from build123d import *

# Parameters (mm, degrees)
SKETCH_1_W      = 16.85
SKETCH_1_H      = 16.85
EXTRUDE_1_DEPTH = 4
SHELL_1_T       = -1.5
FILLET_1_R      = 1


with BuildPart() as part:
    # 草图1 → 凸台-拉伸1 (new body)
    with BuildSketch(Plane(origin=(0, 0, 0), x_dir=(1, 0, 0), z_dir=(0, 1, 0))):
        Rectangle(SKETCH_1_W, SKETCH_1_H)
    extrude(amount=EXTRUDE_1_DEPTH)

    # 抽壳1
    shell_1_openings = [part.faces().sort_by_distance(p)[0] for p in [
        (0, 0, 0),
    ]]
    offset(amount=SHELL_1_T, openings=shell_1_openings, kind=Kind.INTERSECTION)

    # 草图2 → 切除-旋转5 (revolve, cut)
    with BuildSketch(Plane.XY):
        with BuildLine():
            Line((0, 164), (0, 3))
            ThreePointArc((0, 3), (80.5, 83.5), (0, 164))
        make_face()
    revolve(axis=Axis((0, 0, 0), (0, 1, 0)), mode=Mode.SUBTRACT)

    # 圆角1
    fillet_1_edges = [part.edges().sort_by_distance(p)[0] for p in [
        (8.425, 1.943314789, 8.425),
        (-8.425, 1.943314789, 8.425),
        (0, 3.442087368, 8.425),
        (-8.425, 1.943314789, -8.425),
        (8.425, 1.943314789, -8.425),
        (0, 3.442087368, -8.425),
        (8.425, 3.553300166, 4.218359953),
        (-8.425, 3.442087368, 0),
    ]]
    fillet(fillet_1_edges, radius=FILLET_1_R)


solid = part.part
For this review, take the finished solid that the model builds, in its own axes (mm). A direction names the side the tool comes from. Give positions to 0.01 mm unless a question says otherwise; leave off trailing zeros. Loops run counter-clockwise (first coordinate to the right, second up) from the corner with the lowest first, then second, coordinate; pieces in that order, holes last.
Item 1: Draft analysis for pull direction X (two halves, no side actions). For faces 1 (the flat face through (6.925, 1, 0)), 2 (the cylindrical face through (-8.14, 1.358, -8.124)), 3 (the flat face through (-8, 0, 0)), 4 (the flat face through (8.425, 1, 0)), state which applies: +X half, -X half, draft (parallel to the pull), parting line (faces both ways), or undercut.
Item 2: Tool access review of faces 5 (the flat face through (-6.925, 1, 0)), 6 (the flat face through (0, 1, -8.425)): name each direction out of +Z, -Z, +X, -X, +Y, -Y from which nothing blocks a thin tool from reaching the whole face with its end or side.
Item 3: Insertion check: pin 1 (1 mm diameter, centred on x = 3, z = 2, fed in from -Y); pin 2 (5 mm diameter, centred on x = -2, z = -4.5, fed in from -Y). Each pin has a flat end and moves straight along its axis. Give the tip position at first contact, or say it passes through.
Item 4: Take a section at A-A, the plane y = 0.2. State the section outline as (x, z) points (3 decimals), and give its area (3 significant figures).
Item 5: For line 1 along Z through (x, y) = (-1.75, 1.25) (3 decimals); line 2 along X through (y, z) = (2.55, -5), list the stretches that pass through material, from the lowest coordinate up.
Calculated:
1. face 1: undercut
1. face 2: -X half
1. face 3: draft
1. face 4: +X half
2. face 5: -Y
2. face 6: -Z, +X, -X, +Y, -Y
3. pin 1: stops at y = 2.5
3. pin 2: stops at y = 0
4. outline: (-8.425, -7.425) arc R1 ccw to (-7.425, -8.425) - (7.425, -8.425) arc R1 ccw to (8.425, -7.425) - (8.425, 7.425) arc R1 ccw to (7.425, 8.425) - (-7.425, 8.425) arc R1 ccw to (-8.425, 7.425) - close; hole (-6.925, -6.925) - (6.925, -6.925) - (6.925, 6.925) - (-6.925, 6.925) - close
4. area: 91.2 mm2
5. line 1: z = -8.425 to -6.925, 6.925 to 8.425
5. line 2: x = -8.42 to 8.42
